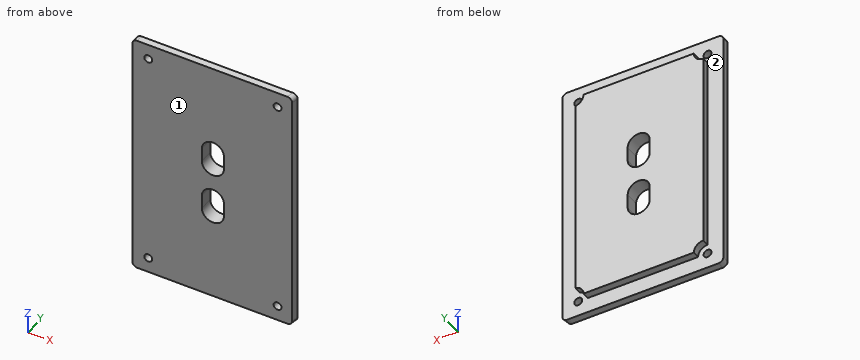
Autodesk Inventor part; units mm, degrees
ref_plane "YZ Plane" through (0, 0, 0) normal (1, 0, 0) x (0, 1, 0)
ref_plane "XZ Plane" through (0, 0, 0) normal (0, 1, 0) x (-1, 0, 0)
ref_plane "XY Plane" through (0, 0, 0) normal (0, 0, 1) x (1, 0, 0)
sketch "Esboço1" plane through (0, 0, 0) normal (0, 1, 0) x (-1, 0, 0)
  line L0 (-34, 53) -> (34, 53)
  line L1 (34, 53) -> (34, -53)
  line L2 (34, -53) -> (-34, -53)
  line L3 (-34, -53) -> (-34, 53)
  line L4 (-34, 53) -> (34, -53) construction
  line L5 (34, 53) -> (-34, -53) construction
  point P0 (0, 0)
  dimension "d0" = 68
  dimension "d1" = 106
extrude "Extrusão1" add sketch "Esboço1" along normal blind 3
sketch "Esboço4" plane through (0, 3, 0) normal (0, 1, 0) x (1, 0, 0)
  line L0 (29.972, -49.0345) -> (-29.972, -49.0345)
  line L1 (-29.972, -49.0345) -> (-29.972, 49.0345)
  line L2 (-29.972, 49.0345) -> (29.972, 49.0345)
  line L3 (29.972, 49.0345) -> (29.972, -49.0345)
  line L4 (29.972, -49.0345) -> (-29.972, 49.0345) construction
  line L5 (-29.972, -49.0345) -> (29.972, 49.0345) construction
  circle A0 centre (-27.305, -46.4815) radius 1.6765
  circle A1 centre (27.305, -46.4815) radius 1.6765
  circle A2 centre (-27.305, 46.4825) radius 1.6765
  circle A3 centre (27.305, 46.4825) radius 1.6765
  point P0 (0, 0)
  dimension "d11" = 59.944
  dimension "d12" = 98.069
  dimension "d13" = 3.353
  dimension "d14" = 2.667
  dimension "d15" = 2.553
  dimension "d18" = 54.61
  dimension "d21" = 92.964
extrude "Extrusão3" cut sketch "Esboço4" against normal blind 3 contours A0 | A1 | A2 | A3
sketch "Esboço5" plane through (0, 3, 0) normal (0, 1, 0) x (1, 0, 0)
  circle A0 centre (-27.305, -46.4815) radius 1.6765
  arc A1 (-23.305, -46.4825) -> (-27.305, -42.4815) centre (-27.305, -46.4815) ccw
  circle A2 centre (27.305, -46.4815) radius 1.6765
  arc A3 (26.645, -42.5363) -> (23.305, -46.4825) centre (27.305, -46.4815) ccw
  circle A4 centre (27.305, 46.4825) radius 1.6765
  arc A5 (23.305, 46.4825) -> (26.645, 42.5373) centre (27.305, 46.4825) ccw
  circle A6 centre (-27.305, 46.4825) radius 1.6765
  arc A7 (-27.305, 42.4825) -> (-23.305, 46.4825) centre (-27.305, 46.4825) ccw
  line L0 (26.645, 42.5373) -> (26.645, -42.5363)
  line L1 (27.1364, -46.1956) -> (-27.305, 46.4825) construction
  line L2 (-26.975, -46.4825) -> (26.975, 46.4825) construction
  line L3 (-27.305, -42.4815) -> (-27.305, 42.4825)
  line L4 (23.305, -46.4825) -> (-23.305, -46.4825)
  line L5 (-23.305, 46.4825) -> (23.305, 46.4825)
  point P0 (0, 0)
  dimension "d26" = 8
  dimension "d27" = 8
  dimension "d28" = 8
  dimension "d29" = 8
extrude "Extrusão4" add sketch "Esboço5" along normal blind 3 contours A1 L3 A7 L5 A5 L0 A3 L4
sketch "Esboço7" plane through (-34, 0, 53) normal (0, 0, 1) x (1, 0, 0)
  line L0 (68, 0) -> (68, 3)
  line L1 (68, 0) -> (68, 3)
  line L2 (68, 3) -> (67.4537, -0.098)
  line L3 (67.4537, -0.098) -> (68, -0.098)
  line L4 (68, 0) -> (0, 0)
  line L5 (68, -0.098) -> (68, 0)
  line L6 (68, 3) -> (0, 3)
  line L7 (68, 0) -> (68, 3)
  point P0 (34, 0)
  dimension "d36" = 10
extrude "Extrusão6" cut sketch "Esboço7" against normal blind 114
fillet "Arredondamento1" radius 2 4 edges at (-34, 1.5, 53) (33.7355, 1.5, 53) (-34, 1.5, -53) (33.7355, 1.5, -53)
sketch "Esboço8" plane through (0, 6, 0) normal (0, 1, 0) x (1, 0, 0)
  arc A0 (4.65, 14) -> (-4.65, 14) centre (0, 14) ccw
  arc A1 (-4.65, 8) -> (4.65, 8) centre (0, 8) ccw
  arc A2 (4.65, -8) -> (-4.65, -8) centre (0, -8) ccw
  arc A3 (-4.65, -14) -> (4.65, -14) centre (0, -14) ccw
  line L0 (4.65, 14) -> (4.65, 8)
  line L1 (-4.65, 14) -> (-4.65, 8)
  line L2 (4.65, -8) -> (4.65, -14)
  line L3 (-4.65, -14) -> (-4.65, -8)
  point P0 (0, 0)
  dimension "d40" = 9.3
  dimension "d41" = 9.3
  dimension "d42" = 9.3
  dimension "d43" = 9.3
  dimension "d44" = 6
  dimension "d45" = 6
  dimension "d46" = 8
  dimension "d47" = 8
extrude "Extrusão7" cut sketch "Esboço8" against normal blind 10
properties part number "tampa"
Geometry check sheet. Reference: the model listing, model coordinates, mm. Face numbers are marked on the shaded views. A direction names the side the tool comes from. Round coordinates to 2 decimals unless told otherwise and drop trailing zeros. Loops run counter-clockwise (first coordinate to the right, second up) from the corner with the lowest first, then second, coordinate; pieces in that order, holes last. Notation, with made-up numbers: (3, -27) - (52, -27) arc R31 cw to (52, 8) - close; hole circle Ø9 at (-27.75, -1.75). An arc over 180 degrees is marked (long way). Answer as CSV lines item,"result".
(1) Cross-section at B-B, the plane z = -1. Enter the section's corners in (x, y) (3 decimals).
Output values:
outline,"(-34, 0) - (33.471, 0) - (34, 3) - (26.645, 3) - (26.645, 6) - (-27.305, 6) - (-27.305, 3) - (-34, 3) - close"
(2) Cross-section at A-A, the plane x = 0. Enter the section's corners in (y, z).
Output values:
outline,"(0, -53) - (3, -53) - (3, -46.48) - (6, -46.48) - (6, -18.65) - (0, -18.65) - close; (0, -3.35) - (6, -3.35) - (6, 3.35) - (0, 3.35) - close; (0, 18.65) - (6, 18.65) - (6, 46.48) - (3, 46.48) - (3, 53) - (0, 53) - close"
(3) Cross-section at D-D, the plane y = 1.15. Give the number of separate pieces and of enclosed holes in the cut face, and give its area (3 significant figures).
Output values:
separate pieces,"1"
enclosed holes,"6"
area,"6,890 mm²"
(4) Material ranges on line 1 along Z through (x, y) = (2, 4.55); line 2 along Z through (x, y) = (-0.5, 3.6); line 3 along Z through (x, y) = (-22, 3.95), recorded low to high.
Output values:
line 1,"z = -46.48 to -18.2, -3.8 to 3.8, 18.2 to 46.48"
line 2,"z = -46.48 to -18.62, -3.38 to 3.38, 18.62 to 46.48"
line 3,"z = -46.48 to 46.48"
(5) Cross-section at C-C, the plane x = 11. Enter the section's corners in (y, z).
Output values:
outline,"(0, -53) - (3, -53) - (3, -46.48) - (6, -46.48) - (6, 46.48) - (3, 46.48) - (3, 53) - (0, 53) - close"
(6) Set-up check for the marked faces 1 and 2: record each of +Z, -Z, +X, -X, +Y, -Y from which the full face is reachable in a straight line by a thin tool's end or side.
Output values:
face 1,"+Z, -Z, +X, -X, -Y"
face 2,"+Y"
(7) Depth check by flat-ended pin: pin 1 Ø2.5 at (y, z) = (4, -3.5) entering from -X; pin 2 Ø3.5 at (y, z) = (5, -10) entering from +X (3 decimals); pin 3 Ø1 at (y, z) = (2, 25.5) entering from +X; pin 4 Ø5.5 at (x, z) = (27.3, 46.48) entering from +Y. Enter the tip coordinate at first touch or a pass-through.
Output values:
pin 1,"stops at x = -34"
pin 2,"stops at x = 26.645"
pin 3,"stops at x = 33.91"
pin 4,"stops at y = 3"
